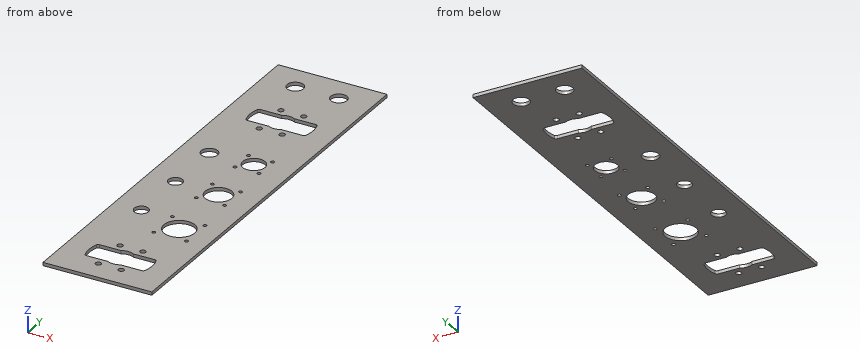
```python
from build123d import *

# Parameters (mm, degrees)
SKETCH1_W           = 100
SKETCH1_H           = 380
BOSS_EXTRUDE1_DEPTH = 3
SKETCH1_3_R         = 6.5
SKETCH1_3_R_2       = 7.5
SKETCH1_3_R_3       = 2.6
SKETCH1_3_R_4       = 1.6
SKETCH1_3_R_5       = 14.25
SKETCH1_3_R_6       = 12.25
SKETCH1_3_R_7       = 10.25
CUT_EXTRUDE1_DEPTH  = 3


with BuildPart() as part:
    # Sketch1 → Boss-Extrude1 (new body)
    with BuildSketch(Plane.XY):
        with Locations((50, 190)):
            Rectangle(SKETCH1_W, SKETCH1_H)
    extrude(amount=-BOSS_EXTRUDE1_DEPTH)

    # Sketch1<3> → Cut-Extrude1 (cut)
    with BuildSketch(Plane.XY):
        with Locations((25, 170)):
            Circle(SKETCH1_3_R)
        with Locations((25, 115)):
            Circle(SKETCH1_3_R)
        with Locations((25, 225)):
            Circle(SKETCH1_3_R_2)
        with Locations((70, 355)):
            Circle(SKETCH1_3_R_2)
        with Locations((30, 355)):
            Circle(SKETCH1_3_R_2)
        with Locations((39.5, 20)):
            Circle(SKETCH1_3_R_3)
        with Locations((60.5, 20)):
            Circle(SKETCH1_3_R_3)
        with Locations((39.5, 55)):
            Circle(SKETCH1_3_R_3)
        with Locations((60.5, 55)):
            Circle(SKETCH1_3_R_3)
        with Locations((39.5, 280)):
            Circle(SKETCH1_3_R_3)
        with Locations((60.5, 280)):
            Circle(SKETCH1_3_R_3)
        with Locations((39.5, 315)):
            Circle(SKETCH1_3_R_3)
        with Locations((60.5, 315)):
            Circle(SKETCH1_3_R_3)
        with Locations((52, 117.5)):
            Circle(SKETCH1_3_R_4)
        with Locations((82, 117.5)):
            Circle(SKETCH1_3_R_4)
        with Locations((52, 87.5)):
            Circle(SKETCH1_3_R_4)
        with Locations((82, 87.5)):
            Circle(SKETCH1_3_R_4)
        with Locations((67, 102.5)):
            Circle(SKETCH1_3_R_5)
        with Locations((66, 167.5)):
            Circle(SKETCH1_3_R_6)
        with Locations((53, 180.5)):
            Circle(SKETCH1_3_R_4)
        with Locations((79, 180.5)):
            Circle(SKETCH1_3_R_4)
        with Locations((79, 154.5)):
            Circle(SKETCH1_3_R_4)
        with Locations((53, 154.5)):
            Circle(SKETCH1_3_R_4)
        with Locations((65.5, 225.5)):
            Circle(SKETCH1_3_R_7)
        with Locations((54.5, 236.5)):
            Circle(SKETCH1_3_R_4)
        with Locations((76.5, 236.5)):
            Circle(SKETCH1_3_R_4)
        with Locations((54.5, 214.5)):
            Circle(SKETCH1_3_R_4)
        with Locations((76.5, 214.5)):
            Circle(SKETCH1_3_R_4)
        with BuildLine():
            Line((44.190524981, 48), (24.478244574, 48))
            ThreePointArc((24.478244574, 48), (23.30861654, 47.622334818), (22.58071629, 46.63197026))
            ThreePointArc((22.58071629, 46.63197026), (21.1, 37.5), (22.58071629, 28.36802974))
            ThreePointArc((22.58071629, 28.36802974), (23.30861654, 27.377665182), (24.478244574, 27))
            Line((24.478244574, 27), (44.190524981, 27))
            ThreePointArc((44.190524981, 27), (50, 25.5), (55.809475019, 27))
            Line((55.809475019, 27), (75.521755425, 27))
            ThreePointArc((75.521755425, 27), (76.69138346, 27.377665182), (77.41928371, 28.36802974))
            ThreePointArc((77.41928371, 28.36802974), (78.9, 37.5), (77.41928371, 46.63197026))
            ThreePointArc((77.41928371, 46.63197026), (76.69138346, 47.622334818), (75.521755426, 48))
            Line((75.521755426, 48), (55.809475019, 48))
            ThreePointArc((55.809475019, 48), (50, 49.5), (44.190524981, 48))
        make_face()
        with BuildLine():
            Line((44.190524981, 308), (24.478244574, 308))
            ThreePointArc((24.478244574, 308), (23.30861654, 307.622334818), (22.58071629, 306.63197026))
            ThreePointArc((22.58071629, 306.63197026), (21.1, 297.5), (22.58071629, 288.36802974))
            ThreePointArc((22.58071629, 288.36802974), (23.30861654, 287.377665182), (24.478244574, 287))
            Line((24.478244574, 287), (44.190524981, 287))
            ThreePointArc((44.190524981, 287), (50, 285.5), (55.809475019, 287))
            Line((55.809475019, 287), (75.521755426, 287))
            ThreePointArc((75.521755426, 287), (76.69138346, 287.377665182), (77.41928371, 288.36802974))
            ThreePointArc((77.41928371, 288.36802974), (78.9, 297.5), (77.41928371, 306.63197026))
            ThreePointArc((77.41928371, 306.63197026), (76.69138346, 307.622334818), (75.521755426, 308))
            Line((75.521755426, 308), (55.809475019, 308))
            ThreePointArc((55.809475019, 308), (50, 309.5), (44.190524981, 308))
        make_face()
    extrude(amount=-CUT_EXTRUDE1_DEPTH, mode=Mode.SUBTRACT)


solid = part.part
```
Geometry check sheet. Reference: the model listing, model coordinates, mm. Coordinates: 2 decimals unless noted, no trailing zeros. Loops run counter-clockwise (first coordinate to the right, second up) from the corner with the lowest first, then second, coordinate; pieces in that order, holes last.
Item 1: Sectioned sample at A-A, the plane y = 355. Record the boundary of the cut face in (x, z), then the cut area to 3 significant figures.
Item 2: Go/stop test with a flat-tipped pin: pin 1 Ø12 at (x, y) = (25, 225) entering from +Z. Record where the tip stops, or that it passes through.
Item 3: Sectioned sample at C-C, the plane x = 69. Record the boundary of the cut face in (y, z).
Item 4: Sectioned sample at B-B, the plane y = 102.5. Record the boundary of the cut face in (x, z), then the cut area to 4 significant figures.
Item 5: Thickness scan on line 1 (Y direction, x = 82, z = -2.2); line 2 (X direction, y = 87.5, z = -0.95); line 3 (X direction, y = 154.5, z = -2.3). Record the ranges inside material, lowest first.
Check result:
1. outline: (0, -3) - (22.5, -3) - (22.5, 0) - (0, 0) - close; (37.5, -3) - (62.5, -3) - (62.5, 0) - (37.5, 0) - close; (77.5, -3) - (100, -3) - (100, 0) - (77.5, 0) - close
1. area: 210 mm2
2. pin 1: passes through
3. outline: (0, -3) - (27, -3) - (27, 0) - (0, 0) - close; (48, -3) - (88.39, -3) - (88.39, 0) - (48, 0) - close; (116.61, -3) - (155.62, -3) - (155.62, 0) - (116.61, 0) - close; (179.38, -3) - (215.87, -3) - (215.87, 0) - (179.38, 0) - close; (235.13, -3) - (287, -3) - (287, 0) - (235.13, 0) - close; (308, -3) - (347.57, -3) - (347.57, 0) - (308, 0) - close; (362.43, -3) - (380, -3) - (380, 0) - (362.43, 0) - close
4. outline: (0, -3) - (52.75, -3) - (52.75, 0) - (0, 0) - close; (81.25, -3) - (100, -3) - (100, 0) - (81.25, 0) - close
4. area: 214.5 mm2
5. line 1: y = 0 to 85.9, 89.1 to 115.9, 119.1 to 380
5. line 2: x = 0 to 50.4, 53.6 to 80.4, 83.6 to 100
5. line 3: x = 0 to 51.4, 54.6 to 77.4, 80.6 to 100
